Autodesk Inventor part; units mm, degrees
ref_plane "YZ Plane" through (0, 0, 0) normal (1, 0, 0) x (0, 1, 0)
ref_plane "XZ Plane" through (0, 0, 0) normal (0, 1, 0) x (-1, 0, 0)
ref_plane "XY Plane" through (0, 0, 0) normal (0, 0, 1) x (1, 0, 0)
sketch "Sketch1" plane through (0, 0, 0) normal (1, 0, 0) x (0, 1, 0)
  arc A0 (13.0108, -7.4161) -> (-14.976, 0) centre (0, 0) ccw
  arc A1 (-14.976, -44) -> (-2.6118, -45.5074) centre (-8.702, -44) ccw
  arc A2 (2.4963, -25.8629) -> (1.8506, -27.478) centre (8, -29) ccw
  line L0 (0, -65.4344) -> (0, 32.8066)
  line L1 (1.8506, -27.478) -> (-2.6118, -45.5074)
  line L2 (13.0108, -7.4161) -> (2.4963, -25.8629)
  line L3 (-14.976, 0) -> (-14.976, -44)
  arc A3 (13.3375, -7.6023) -> (-15.352, 0) centre (0, 0) ccw
  line L4 (13.3375, -7.6023) -> (2.8229, -26.0491)
  arc A4 (2.8229, -26.0491) -> (2.2155, -27.5683) centre (8, -29) ccw
  line L5 (2.2155, -27.5683) -> (-2.2468, -45.5977)
  arc A5 (-15.352, -44) -> (-2.2468, -45.5977) centre (-8.702, -44) ccw
  line L6 (-15.352, -44) -> (-15.352, 0)
  dimension "d0" = 29.952
  dimension "d1" = 12.548
  dimension "d2" = 12.67
  dimension "d3" = 29
  dimension "d4" = 44
  dimension "d5" = 8.702
  dimension "d6" = 8
  dimension "d7" = 0.376
extrude "Extrusion1" add sketch "Sketch1" along normal mid plane 6 contours A0 L0 A3 L4 A4 L5 L1 A2 L2 | A0 L3 A1 L1 L0 L5 A5 L6 A3
properties part number "czesc2paska" material "Rubber"
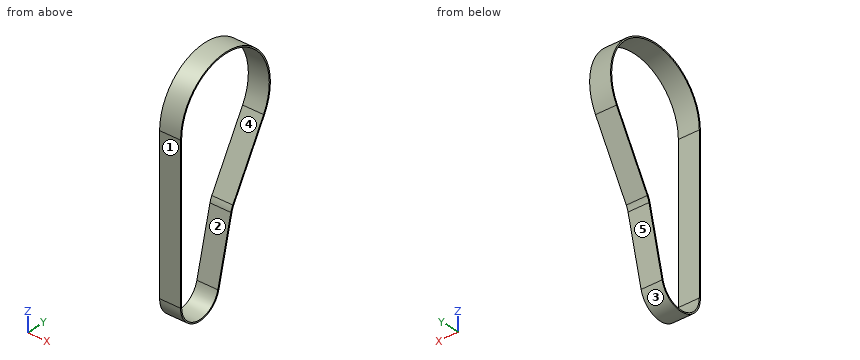
Check sheet for the modelled part. Datum: model origin and axes. Units: mm. Face numbers are marked on the shaded views. A direction names the side the tool comes from. Coordinates: 2 decimals unless noted, no trailing zeros. Loops run counter-clockwise (first coordinate to the right, second up) from the corner with the lowest first, then second, coordinate; pieces in that order, holes last.
1) Gauge pin test, flat ends, axial feed: pin 1 (1 mm diameter, centred on x = 0, y = -2.5, fed in from +Z); pin 2 (1 mm diameter, centred on x = 2.5, y = 2, fed in from +Z). Record the tip position at first contact, or that the pin passes through.
2) Release check for a two-part mould opening along Y. For the marked faces 3, 4 and 5 record: released by +Y, released by -Y, zero draft, split by the parting line, or undercut.
3) Material ranges on probe 1 along Y at (x, z) = (2.6, -41); probe 2 along Y at (x, z) = (-1.25, -11); probe 3 along Z at (x, y) = (0.6, 12.5), recorded low to high.
4) Sectioned sample at A-A (x = -1.25). Record the boundary of the cut face in (y, z).
5) Sectioned sample at B-B (y = -9.5). Record the boundary of the cut face in (x, z).
6) Access from +Z, -Z, +X, -X, +Y, -Y to the whole of each face (thin tool, end or side, straight path). Record for the marked faces 1 and 2.
7) Sectioned sample at C-C (z = -17). Record the boundary of the cut face in (x, y), and give its area (3 significant figures).
Check sheet entries:
1. pin 1: stops at z = 15.22
1. pin 2: stops at z = 15.28
2. face 3: split by the parting line
2. face 4: undercut
2. face 5: released by +Y
3. probe 1: y = -15.35 to -14.98, -1.5 to -1.11
3. probe 2: y = -15.35 to -14.98, 10.97 to 11.4
3. probe 3: z = -9.07 to -8.31, 8.25 to 8.91
4. outline: (-15.35, -44) arc R6.65 ccw to (-2.25, -45.6) - (2.22, -27.57) arc R5.96 cw to (2.82, -26.05) - (13.34, -7.6) arc R15.35 ccw (long way) to (-15.35, 0) - close; hole (-14.98, -44) arc R6.27 ccw to (-2.61, -45.51) - (1.85, -27.48) arc R6.33 cw to (2.5, -25.86) - (13.01, -7.42) arc R14.98 ccw (long way) to (-14.98, 0) - close
5. outline: (-3, -50.6) - (3, -50.6) - (3, -50.22) - (-3, -50.22) - close; (-3, 11.58) - (3, 11.58) - (3, 12.06) - (-3, 12.06) - close
6. face 1: +Z, -Z, +X, -X, -Y
6. face 2: +X, -X
7. outline: (-3, -15.35) - (3, -15.35) - (3, -14.98) - (-3, -14.98) - close; (-3, 7.55) - (3, 7.55) - (3, 7.98) - (-3, 7.98) - close
7. area: 4.85 mm2
